Input: part model. Units: mm. Frame: model coordinates. Coordinates: 2 decimals unless noted, no trailing zeros. Loops run counter-clockwise (first coordinate to the right, second up) from the corner with the lowest first, then second, coordinate; pieces in that order, holes last. Notation, with made-up numbers: (51.5, -13.5) - (82.5, -13.5) arc R25 ccw to (82.5, 3.5) - close; hole circle Ø8 at (55.25, 57.25). An arc over 180 degrees is marked (long way). Write item = value, one per line. Start each with the question number.
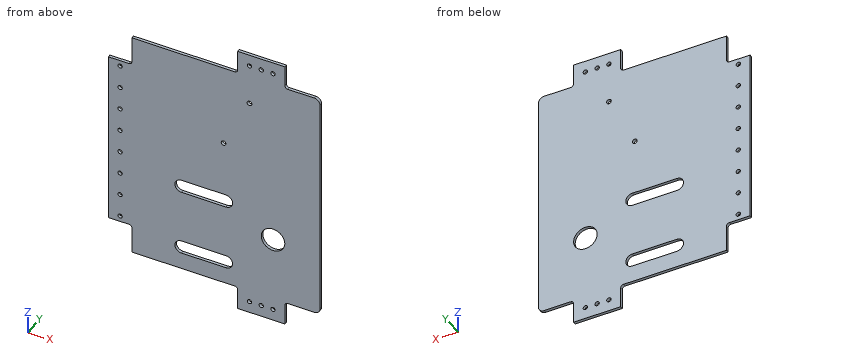
Autodesk Inventor part; units mm, degrees
ref_plane "YZ Plane" through (0, 0, 0) normal (1, 0, 0) x (0, 1, 0)
ref_plane "XZ Plane" through (0, 0, 0) normal (0, 1, 0) x (-1, 0, 0)
ref_plane "XY Plane" through (0, 0, 0) normal (0, 0, 1) x (1, 0, 0)
sketch "Sketch1" plane through (0, 0, 0) normal (0, 1, 0) x (-1, 0, 0)
  line L0 (-38.1, -25.4) -> (-38.1, -279.4)
  line L1 (0, -304.8) -> (50.8, -304.8)
  line L2 (50.8, -304.8) -> (50.8, -279.4)
  line L3 (50.8, -279.4) -> (190.5, -279.4)
  line L4 (190.5, -279.4) -> (190.5, -25.4)
  line L5 (190.5, -25.4) -> (50.8, -25.4)
  line L6 (50.8, -25.4) -> (50.8, 0)
  line L7 (50.8, 0) -> (0, 0)
  circle A0 centre (38.1, -12.7) radius 2.3622
  circle A1 centre (25.4, -12.7) radius 2.3622
  circle A2 centre (12.7, -12.7) radius 2.3622
  line L8 (-38.1, -152.4) -> (190.5, -152.4) construction
  circle A3 centre (177.8, -139.7) radius 2.3622
  circle A4 centre (177.8, -114.3) radius 2.3622
  circle A5 centre (177.8, -88.9) radius 2.3622
  circle A6 centre (177.8, -63.5) radius 2.3622
  circle A7 centre (38.1, -292.1) radius 2.3622
  circle A8 centre (25.4, -292.1) radius 2.3622
  circle A9 centre (12.7, -292.1) radius 2.3622
  circle A10 centre (177.8, -165.1) radius 2.3622
  circle A11 centre (177.8, -190.5) radius 2.3622
  circle A12 centre (177.8, -215.9) radius 2.3622
  circle A13 centre (177.8, -241.3) radius 2.3622
  line L9 (0, 0) -> (0, -25.4)
  line L10 (0, -25.4) -> (-38.1, -25.4)
  line L11 (-38.1, -279.4) -> (0, -279.4)
  line L12 (0, -279.4) -> (0, -304.8)
  line L13 (190.5, -57.15) -> (165.1, -57.15)
  line L14 (165.1, -57.15) -> (165.1, -25.4)
  line L15 (190.5, -247.65) -> (165.1, -247.65)
  line L16 (165.1, -247.65) -> (165.1, -279.4)
  circle A14 centre (66.04, -114.3) radius 2.5527
  circle A15 centre (38.1, -57.15) radius 2.5527
  circle A16 centre (12.7, -209.55) radius 12.7
  circle A17 centre (12.7, -209.55) radius 28.575 construction
  line L17 (111.5, -254) -> (111.5, -182) construction
  line L18 (111.5, -182) -> (63.5, -182) construction
  line L19 (63.5, -182) -> (63.5, -254) construction
  line L20 (63.5, -254) -> (111.5, -254) construction
  line L21 (111.5, -254) -> (63.5, -254) construction
  line L22 (111.5, -246.8562) -> (63.5, -246.8562)
  line L23 (63.5, -261.1437) -> (111.5, -261.1437)
  arc A18 (111.5, -261.1437) -> (111.5, -246.8562) centre (111.5, -254) ccw
  arc A19 (63.5, -246.8562) -> (63.5, -261.1437) centre (63.5, -254) ccw
  line L24 (111.5, -182) -> (63.5, -182) construction
  line L25 (111.5, -174.8562) -> (63.5, -174.8562)
  line L26 (63.5, -189.1437) -> (111.5, -189.1437)
  arc A20 (111.5, -189.1437) -> (111.5, -174.8562) centre (111.5, -182) ccw
  arc A21 (63.5, -174.8562) -> (63.5, -189.1437) centre (63.5, -182) ccw
  point P0 (177.8, -279.4)
  point P1 (120.65, -279.4)
  point P2 (87.5, -254)
  point P3 (87.5, -182)
  dimension "d0" = 254
  dimension "d1" = 50.8
  dimension "d2" = 25.4
  dimension "d4" = 12.7
  dimension "d5" = 12.7
  dimension "d6" = 12.7
  dimension "d7" = 12.7
  dimension "d8" = 4.7244
  dimension "d9" = 12.7
  dimension "d10" = 12.7
  dimension "d13" = 25.4
  dimension "d20" = 228.6
  dimension "d21" = 38.1
  dimension "d22" = 25.4
  dimension "d23" = 6.35
  dimension "d25" = 5.1054
  dimension "d28" = 57.15
  dimension "d29" = 27.94
  dimension "d31" = 25.4
  dimension "d32" = 57.15
  dimension "d33" = 152.4
  dimension "d34" = 69.85
  dimension "d35" = 72
  dimension "d36" = 48
  dimension "d37" = 14.2875
  dimension "d38" = 14.2875
  dimension "d42" = 38.1
  dimension "d43" = 31.75
  dimension "d44" = 0
  dimension "d45" = 25.4
  dimension "d46" = 63.5
extrude "Extrusion1" add sketch "Sketch1" along normal blind 3.175 contours L10 L9 L7 L6 L5 L14 L13 L4 L15 L16 L3 L2 L1 L12 L11 L0
fillet "Fillet1" radius 3.175 6 edges at (-165.1, 1.5875, -57.15) (-165.1, 1.5875, -247.65) (-50.8, 1.5875, -279.4) (0, 1.5875, -279.4) (0, 1.5875, -25.4) (-50.8, 1.5875, -25.4)
fillet "Fillet2" radius 6.35 2 edges at (38.1, 1.5875, -25.4) (38.1, 1.5875, -279.4)
sketch "Cut Sketch" plane through (0, 3.175, 0) normal (0, 1, 0) x (1, 0, 0)
  arc A0 (38.1, 273.05) -> (31.75, 279.4) centre (31.75, 273.05) ccw
  line L0 (31.75, 279.4) -> (3.175, 279.4)
  arc A1 (0, 282.575) -> (3.175, 279.4) centre (3.175, 282.575) ccw
  line L1 (0, 282.575) -> (0, 304.8)
  line L2 (0, 304.8) -> (-50.8, 304.8)
  line L3 (-50.8, 304.8) -> (-50.8, 282.575)
  arc A2 (-53.975, 279.4) -> (-50.8, 282.575) centre (-53.975, 282.575) ccw
  line L4 (-53.975, 279.4) -> (-165.1, 279.4)
  line L5 (-165.1, 279.4) -> (-165.1, 250.825)
  arc A3 (-168.275, 247.65) -> (-165.1, 250.825) centre (-168.275, 250.825) ccw
  line L6 (-168.275, 247.65) -> (-190.5, 247.65)
  line L7 (-190.5, 247.65) -> (-190.5, 57.15)
  line L8 (-190.5, 57.15) -> (-168.275, 57.15)
  arc A4 (-165.1, 53.975) -> (-168.275, 57.15) centre (-168.275, 53.975) ccw
  line L9 (-165.1, 53.975) -> (-165.1, 25.4)
  line L10 (-165.1, 25.4) -> (-53.975, 25.4)
  arc A5 (-50.8, 22.225) -> (-53.975, 25.4) centre (-53.975, 22.225) ccw
  line L11 (-50.8, 22.225) -> (-50.8, 0)
  line L12 (-50.8, 0) -> (0, 0)
  line L13 (0, 0) -> (0, 22.225)
  arc A6 (3.175, 25.4) -> (0, 22.225) centre (3.175, 22.225) ccw
  line L14 (3.175, 25.4) -> (31.75, 25.4)
  arc A7 (31.75, 25.4) -> (38.1, 31.75) centre (31.75, 31.75) ccw
  line L15 (38.1, 31.75) -> (38.1, 273.05)
  circle A8 centre (-12.7, 209.55) radius 12.7
  circle A9 centre (-66.04, 114.3) radius 2.5527
  circle A10 centre (-25.4, 292.1) radius 2.3622
  circle A11 centre (-177.8, 165.1) radius 2.3622
  circle A12 centre (-177.8, 215.9) radius 2.3622
  circle A13 centre (-177.8, 63.5) radius 2.3622
  circle A14 centre (-177.8, 88.9) radius 2.3622
  circle A15 centre (-177.8, 114.3) radius 2.3622
  circle A16 centre (-177.8, 139.7) radius 2.3622
  circle A17 centre (-12.7, 12.7) radius 2.3622
  circle A18 centre (-25.4, 12.7) radius 2.3622
  circle A19 centre (-38.1, 12.7) radius 2.3622
  circle A20 centre (-177.8, 241.3) radius 2.3622
  circle A21 centre (-177.8, 190.5) radius 2.3622
  circle A22 centre (-38.1, 292.1) radius 2.3622
  circle A23 centre (-12.7, 292.1) radius 2.3622
  circle A24 centre (-38.1, 57.15) radius 2.5527
  arc A25 (-111.5, 189.1437) -> (-111.5, 174.8562) centre (-111.5, 182) ccw
  line L16 (-111.5, 189.1437) -> (-63.5, 189.1437)
  arc A26 (-63.5, 174.8562) -> (-63.5, 189.1437) centre (-63.5, 182) ccw
  line L17 (-63.5, 174.8562) -> (-111.5, 174.8562)
  arc A27 (-111.5, 261.1437) -> (-111.5, 246.8562) centre (-111.5, 254) ccw
  line L18 (-111.5, 261.1437) -> (-63.5, 261.1437)
  arc A28 (-63.5, 246.8562) -> (-63.5, 261.1437) centre (-63.5, 254) ccw
  line L19 (-63.5, 246.8562) -> (-111.5, 246.8562)
properties part number "1561 Daughter Board"
Item 1: Pin query (flat end, axial travel): pin 1 (3 mm diameter, centred on x = -177.8, z = -190.5, fed in from +Y); pin 2 (1.6 mm diameter, centred on x = -93, y = 1, fed in from +Z); pin 3 (1.6 mm diameter, centred on x = 24, y = 1, fed in from -Z); pin 4 (1.6 mm diameter, centred on x = -182, y = 2, fed in from +Z). Return the tip coordinate at first contact, or that it passes through.
Item 2: Cut plane B-B on x = -7. Return loops of the section in (y, z) (3 decimals).
Item 3: Cut plane C-C on y = 1.9. State how many separate pieces and enclosed holes the cut face has, plus the area to 3 significant figures.
Item 4: Ray query, line 1 (Z direction, x = -12.7, y = 2.1); line 2 (Z direction, x = -78, y = 0.65); line 3 (X direction, y = 0.75, z = -190.5). Return the intervals inside material, ascending.
Item 5: Cut plane A-A on x = -91. Return loops of the section in (y, z) (3 decimals).
Item 6: Cut plane D-D on z = -46. Return loops of the section in (x, y) (3 decimals).
Recorded:
q1.pin_1 = through
q1.pin_2 = -25.4
q1.pin_3 = -279.4
q1.pin_4 = -57.15
q2.outline = (0, -304.8) - (3.175, -304.8) - (3.175, -220.899) - (0, -220.899) - close; (0, -198.201) - (3.175, -198.201) - (3.175, 0) - (0, 0) - close
q3.separate_pieces = 1
q3.enclosed_holes = 19
q3.area = 56,500 mm²
q4.line_1 = -304.8 to -294.46, -289.74 to -222.25, -196.85 to -15.06, -10.34 to 0
q4.line_2 = -279.4 to -261.14, -246.86 to -189.14, -174.86 to -25.4
q4.line_3 = -190.5 to -180.16, -175.44 to 38.1
q5.outline = (0, -279.4) - (3.175, -279.4) - (3.175, -261.144) - (0, -261.144) - close; (0, -246.856) - (3.175, -246.856) - (3.175, -189.144) - (0, -189.144) - close; (0, -174.856) - (3.175, -174.856) - (3.175, -25.4) - (0, -25.4) - close
q6.outline = (-165.1, 0) - (38.1, 0) - (38.1, 3.175) - (-165.1, 3.175) - close
